For this review, take the finished solid that the model builds, in its own axes (mm). A direction names the side the tool comes from. Round coordinates to 2 decimals unless told otherwise and drop trailing zeros. Loops run counter-clockwise (first coordinate to the right, second up) from the corner with the lowest first, then second, coordinate; pieces in that order, holes last. Notation, with made-up numbers: M 17.5,40 L 28.5,40 A14 ccw 28.5,46 Z; hole C 19.25,-36 d4. An arc over 180 degrees is marked long. One line per question, with ' | ' between items. Start each with the question number.
1) We need section C-C (z = 6.75). Give the boundary of the cut face in (x, y).
2) For probe 1 along Y at (x, z) = (8.5, 5.5); probe 2 along Z at (x, y) = (-4.5, 11.65); probe 3 along X at (y, z) = (5.25, 7.75), list the stretches that pass through material, from the lowest coordinate up. Write a range as from..to.
3) We need section D-D (y = 7.5). Give the boundary of the cut face in (x, z), and give its area (3 significant figures).
4) We need section B-B (x = 11). Give the boundary of the cut face in (y, z).
5) For pin 1 Ø1 at (x, z) = (-6, 2.5) entering from -Y; pin 2 Ø3.5 at (y, z) = (6, 5) entering from -X; pin 3 Ø2 at (y, z) = (2, 4) entering from -X, all flat-tipped, find the tip position at first contact; note any pin that passes through.
6) For faces 1 (the face through (13, 9, 10)), 2 (the face through (25, 6, 5)), 3 (the face through (0, 2, 5)), list the 3-axis set-ups (+Z, -Z, +X, -X, +Y, -Y) from which the entire face can be reached by the end or side of a thin tool; tool diameter is ignored.
7) Mouldability with a two-part tool opening along Y and no side actions: class faces 4 (the face through (9, 12.5, 5)), 5 (the face through (13, 9, 0)), 6 (the face through (13, 4, 5)) as pulls with the +Y half, pulls with the -Y half, needs draft (parallel to the pull), parting line crosses it, or undercut.
8) We need section A-A (z = 5). Give the boundary of the cut face in (x, y), and give its area (3 significant figures).
```python
from build123d import *

# Parameters (mm, degrees)
F1_DEPTH = 10
F2_R     = 1.25
F3_DEPTH = 25


with BuildPart() as f1:
    # F0 (on Top) → F1 (new body)
    with BuildSketch(Plane.XY):
        Polygon((0, 4), (0, 0), (29, 0), (29, 12.5), (-11, 12.5), (-11, 8.5), (25, 8.5), (25, 4), align=None)
    extrude(amount=F1_DEPTH)

    # F2 (on face) → F3 (cut)
    with BuildSketch(Plane.XZ.offset(-8.5)):
        with Locations((-4.5, 5)):
            Circle(F2_R)
    extrude(amount=-F3_DEPTH, mode=Mode.SUBTRACT)


solid = f1.part
```
Answers below:
1) outline: M -11,8.5 L 25,8.5 L 25,4 L 0,4 L 0,0 L 29,0 L 29,12.5 L -11,12.5 Z
2) probe 1: 0..4, 8.5..12.5 | probe 2: 0..3.75, 6.25..10 | probe 3: 25..29
3) outline: M 25,0 L 29,0 L 29,10 L 25,10 Z | area: 40.0 mm^2
4) outline: M 0,0 L 4,0 L 4,10 L 0,10 Z; M 8.5,0 L 12.5,0 L 12.5,10 L 8.5,10 Z
5) pin 1: y = 8.5 | pin 2: x = 25 | pin 3: x = 0
6) face 1: +Z, +X, -X, +Y, -Y | face 2: +Z, -Z, -X | face 3: +Z, -Z, -X, -Y
7) face 4: pulls with the +Y half | face 5: needs draft | face 6: undercut
8) outline: M -11,8.5 L -5.75,8.5 L -5.75,12.5 L -11,12.5 Z; M -3.25,8.5 L 25,8.5 L 25,4 L 0,4 L 0,0 L 29,0 L 29,12.5 L -3.25,12.5 Z | area: 284 mm^2
